Model file for the job. Use its own axes, mm. Round coordinates to 2 decimals unless told otherwise and drop trailing zeros. Answer in a Markdown table with one row per item.
from build123d import *

# Parameters (mm, degrees)
F0_R      = 2.667
F0_R_2    = 4.445
F1_DEPTH  = 2.032
F2_R      = 3.81
F2_R_2    = 2.667
F3_DEPTH  = 1.016
F4_R      = 0.8255
F5_DEPTH  = 25.4
F6_R      = 1.27
F6_R_2    = 0.8255
F7_DEPTH  = 1.016
F8_DEPTH  = 1.016
F9_R      = 1.27
F9_R_2    = 0.8255
F9_R_3    = 3.81
F9_R_4    = 2.667
F10_DEPTH = 1.016


with BuildPart() as f1:
    # F0 (on Top) → F1 (new body)
    with BuildSketch(Plane.XY):
        with BuildLine():
            add(Edge.make_bspline(
                [(-145.8688657386, -44.8941665066), (-120.4979013513, -64.0094905591), (-61.2157028163, -69.6417423021), (-14.9939787657, -65.1516662724)],
                knots=[9.1704042636, 9.1704042636, 9.1704042636, 9.1704042636, 137.9629328019, 137.9629328019, 137.9629328019, 137.9629328019], degree=3))
            ThreePointArc((-14.9939787657, -65.1516662724), (-9.3240486247, -58.5746731476), (-15.5187291961, -52.4893729096))
            add(Edge.make_bspline(
                [(-146.219773699, -28.7446715558), (-115.4057267109, -58.8297417696), (-57.5004960396, -57.185757191), (-15.5187291961, -52.4893729096)],
                knots=[0, 0, 0, 0, 132.8404075443, 132.8404075443, 132.8404075443, 132.8404075443], degree=3))
            ThreePointArc((-146.219773699, -28.7446715558), (-153.6835655793, -31.2301073118), (-153.0025163181, -39.0673103865))
            Line((-153.0025163181, -39.0673103865), (-148.6487479934, -42.6235234818))
            Line((-148.6487479934, -42.6235234818), (-145.8688657386, -44.8941665066))
        make_face()
        with BuildLine():
            ThreePointArc((-139.2748018361, -39.2084827255), (-139.1474453557, -39.29610811), (-139.0263023063, -39.3921406184))
            add(Edge.make_bspline(
                [(-139.0263023063, -39.3921406184), (-115.7533807903, -56.4645604087), (-60.1022871914, -61.7792620614), (-26.4109737279, -57.7751529221)],
                knots=[0.4075873512, 0.4075873512, 0.4075873512, 0.4075873512, 114.3528485972, 114.3528485972, 114.3528485972, 114.3528485972], degree=3))
            ThreePointArc((-26.4109737279, -57.7751529221), (-26.3245090015, -57.7631456427), (-26.237648884, -57.754448306))
            ThreePointArc((-26.237648884, -57.754448306), (-23.7748016763, -59.8487204067), (-25.869073777, -62.3115676144))
            add(Edge.make_bspline(
                [(-25.869073777, -62.3115676144), (-50.1594431698, -65.0675445795), (-110.3361174464, -63.282199204), (-141.7372077703, -43.1182831526)],
                knots=[0, 0, 0, 0, 117.4470376107, 117.4470376107, 117.4470376107, 117.4470376107], degree=3))
            ThreePointArc((-141.7372077703, -43.1182831526), (-142.408403822, -39.9652454073), (-139.2748018361, -39.2084827255))
        make_face(mode=Mode.SUBTRACT)
        with Locations((-15.6686027753, -58.8376039948)):
            Circle(F0_R, mode=Mode.SUBTRACT)
        with Locations((-148.3766692678, -34.7171334858)):
            Circle(F0_R_2, mode=Mode.SUBTRACT)
    extrude(amount=F1_DEPTH)

    # F2 (on face) → F3 (cut)
    with BuildSketch(Plane.XY.offset(2.032)):
        with Locations((-15.6686027753, -58.8376039948)):
            Circle(F2_R)
        with Locations((-15.6686027753, -58.8376039948)):
            Circle(F2_R_2, mode=Mode.SUBTRACT)
    extrude(amount=-F3_DEPTH, mode=Mode.SUBTRACT)

    # F4 (on face) → F5 (cut)
    with BuildSketch(Plane.XY.offset(2.032)):
        with Locations((-143.7340378761, -38.8674512506)):
            Circle(F4_R)
    extrude(amount=-F5_DEPTH, mode=Mode.SUBTRACT)

    # F6 (on face) → F7 (cut)
    with BuildSketch(Plane.XY.offset(2.032)):
        with Locations((-143.7340378761, -38.8674512506)):
            Circle(F6_R)
        with Locations((-143.7340378761, -38.8674512506)):
            Circle(F6_R_2, mode=Mode.SUBTRACT)
    extrude(amount=-F7_DEPTH, mode=Mode.SUBTRACT)

    # F8 (add, through all): faces of the model
    f8_faces = [f1.faces().sort_by_distance(p)[0] for p in [
        (-144.9681168516, -38.8674512506, 1.016),
        (-19.3708397018, -58.8376039948, 1.016),
    ]]
    extrude(f8_faces, amount=F8_DEPTH)

    # F9 (on face) → F10 (cut)
    with BuildSketch(Plane(origin=(0, 0, 0), x_dir=(1, 0, 0), z_dir=(0, 0, -1))):
        with Locations((-143.7340378761, 38.8674512506)):
            Circle(F9_R)
        with Locations((-143.7340378761, 38.8674512506)):
            Circle(F9_R_2, mode=Mode.SUBTRACT)
        with Locations((-15.6686027753, 58.8376039948)):
            Circle(F9_R_3)
        with Locations((-15.6686027753, 58.8376039948)):
            Circle(F9_R_4, mode=Mode.SUBTRACT)
    extrude(amount=-F10_DEPTH, mode=Mode.SUBTRACT)


solid = f1.part
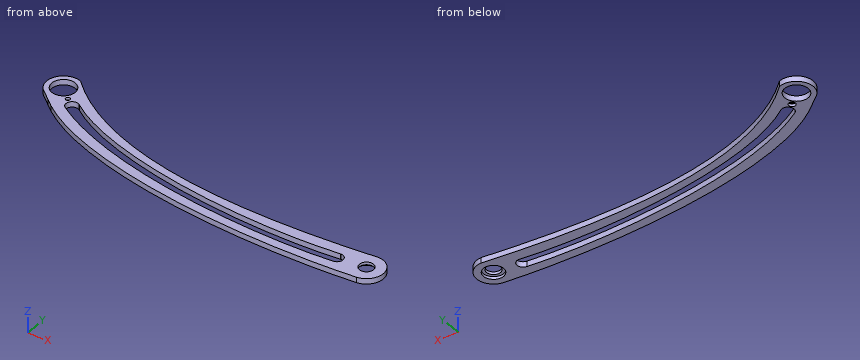
1. Wall check: probe 1 along X at (y, z) = (-38, 0.1); probe 2 along Y at (x, z) = (-92, 1.2); probe 3 along Y at (x, z) = (-122, 0.5). Give the ranges that are in metal, low to high.
Verdict:
| item | result |
|---|---|
| probe 1 | x = -153.81 to -151.37, -145.38 to -144.66, -142.81 to -134.44 |
| probe 2 | y = -63.34 to -59.78, -55.67 to -52.71 |
| probe 3 | y = -56.5 to -52.43, -48.1 to -44.47 |
2. Pin check, flat tips, straight feed: pin 1 (8 mm diameter, centred on x = -42, y = -57, fed in from -Z); pin 2 (1 mm diameter, centred on y = -53.5, z = 1.5, fed in from -X); pin 3 (2 mm diameter, centred on x = -143.73, y = -38.87, fed in from -Z); pin 4 (1 mm diameter, centred on x = -143.73, y = -38.87, fed in from -Z). Stop position of each tip, or through.
Verdict:
| item | result |
|---|---|
| pin 1 | stops at z = 0 |
| pin 2 | stops at x = -131.39 |
| pin 3 | stops at z = 1.02 |
| pin 4 | passes through |
3. Saw through at A-A (z = 1.55). State how many separate pieces and enclosed holes the cut face has, and give its area (3 significant figures).
Verdict:
| item | result |
|---|---|
| separate pieces | 1 |
| enclosed holes | 4 |
| area | 1,110 mm² |
